Answer from the drawing. Dimensions are ordinates in mm from the lowest x, y and z of the part. A direction names the side the tool comes from. Coordinates: 2 decimals unless noted, no trailing zeros. Write each loop counter-clockwise with the first axis right and the second up, starting at its lowest first coordinate (ties: lowest second). Pieces come first, ordered by that corner, then holes. Notation, with made-up numbers: (0, 34.5) -> (46, 34.5) arc R25 cw to (46, 62.5) -> close; hole circle Ø1 at (58.5, 48.5). An arc over 180 degrees is marked (long way). Answer as a JSON object with one key per item and string values. Group by question number.
(1) Find section A-A (x = 17.5). Give the vertices of the cut face in (y, z), then the cut area to 3 significant figures.
(2) Flat-ended cylindrical pins translate along their axes: P1, Ø1.5, axis at x = 17.5, y = 54.5, coming from the +Z side; P2, Ø2, axis at x = 33.5, z = 33, coming from the +Y side; P3, Ø6, axis at x = 15, z = 29, coming from the +Y side. Find the tip coordinate at first contact, or state that the pin passes through.
(3) Find section B-B (z = 21). Give the vertices of the cut face in (x, y).
(4) Find section D-D (z = 5.5). Give the vertices of the cut face in (x, y), then the cut area to 3 significant figures.
(5) Find section C-C (y = 49). Give the vertices of the cut face in (x, z), then the cut area to 3 significant figures.
(6) Straight lines are drawn through the part: L1, parallel to Y at x = 34, z = 6; L2, parallel to Y at x = 23, z = 17; L3, parallel to Z at x = 19, y = 45. For each, find the intervals that lie inside material, in ascending order.
(7) Which of the six approach directions +Z, -Z, +X, -X, +Y, -Y give full straight-line access (tool end or side, diameter ignored) to the marked faces 1 and 2?
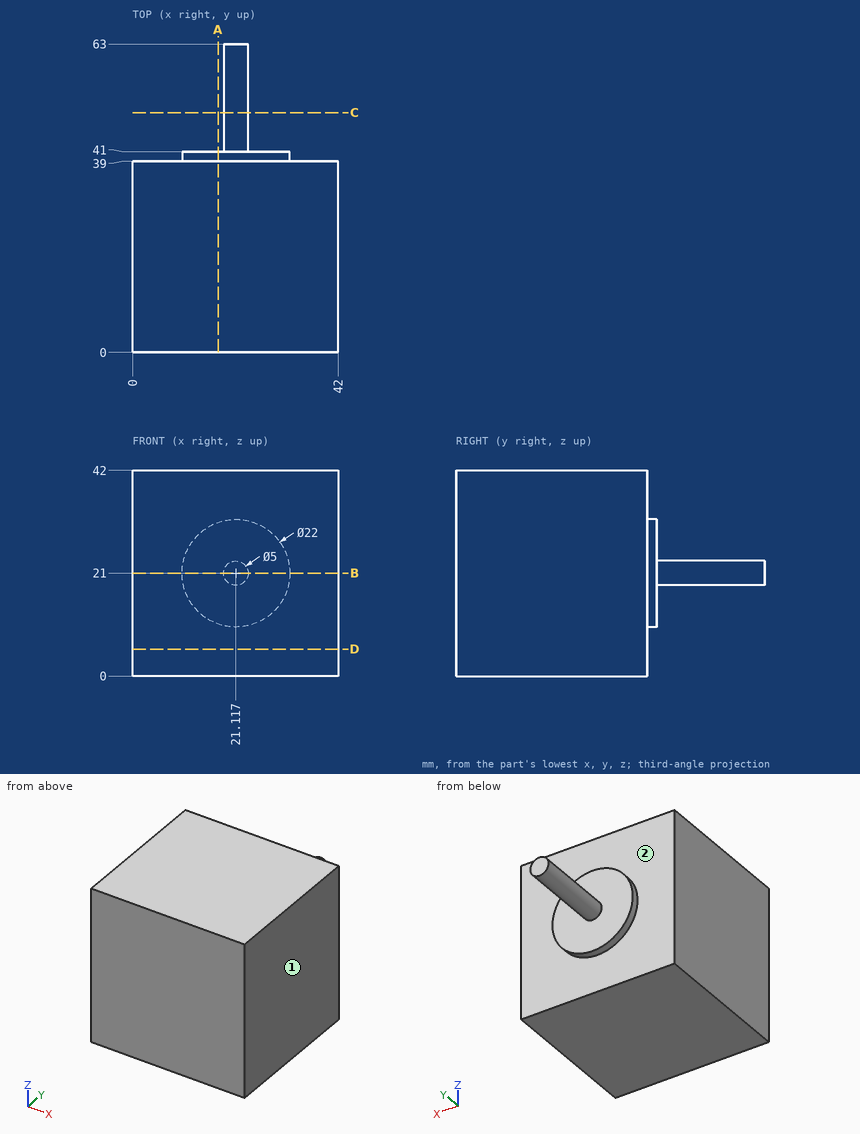
Results below:
{
 "1": {"outline": "(0, 0) -> (39, 0) -> (39, 10.61) -> (41, 10.61) -> (41, 31.39) -> (39, 31.39) -> (39, 42) -> (0, 42) -> close", "area": "1,680 mm2"},
 "2": {"P1": "passes through", "P2": "stops at y = 39", "P3": "stops at y = 41"},
 "3": {"outline": "(0, 0) -> (42, 0) -> (42, 39) -> (32.12, 39) -> (32.12, 41) -> (23.62, 41) -> (23.62, 63) -> (18.62, 63) -> (18.62, 41) -> (10.12, 41) -> (10.12, 39) -> (0, 39) -> close"},
 "4": {"outline": "(0, 0) -> (42, 0) -> (42, 39) -> (0, 39) -> close", "area": "1,640 mm2"},
 "5": {"outline": "circle Ø5 at (21.12, 21)", "area": "19.6 mm2"},
 "6": {"L1": "y = 0 to 39", "L2": "y = 0 to 41", "L3": "z = 19.67 to 22.33"},
 "7": {"face 1": "+Z, -Z, +X, +Y, -Y", "face 2": "+Y"}
}
